from build123d import *

# Parameters (mm, degrees)
SKETCH2_W             = 39.3827
SKETCH2_H             = 7.62
BOSS_EXTRUDE2_DEPTH   = 4.445
BOSS_EXTRUDE2_2_DEPTH = 4.445
BOSS_EXTRUDE3_DEPTH   = 2.54
BOSS_EXTRUDE4_DEPTH   = 44.45
CUT_EXTRUDE3_REACH    = 78.845
SKETCH5_R             = 2.54
SKETCH5_R_2           = 1.0668
CUT_EXTRUDE5_DEPTH    = 41.91
CUT_EXTRUDE7_START    = 2.54
SKETCH7_W             = 22.974442495
SKETCH7_H             = 3.048
CUT_EXTRUDE7_DEPTH    = 16.51
CUT_EXTRUDE8_DEPTH    = 22.974442495


with BuildPart() as part:
    # Sketch2 → Boss-Extrude2 (new body)
    with BuildSketch(Plane(origin=(0, 0, 0), x_dir=(1, 0, 0), z_dir=(0, 1, 0))):
        with Locations((19.69135, 3.81)):
            Rectangle(SKETCH2_W, SKETCH2_H)
    extrude(amount=BOSS_EXTRUDE2_DEPTH)



with BuildPart() as body_2:
    # Sketch2 → Boss-Extrude2 2 (new body)
    with BuildSketch(Plane(origin=(0, 0, 0), x_dir=(1, 0, 0), z_dir=(0, 1, 0))):
        with Locations((19.69135, 72.39)):
            Rectangle(SKETCH2_W, SKETCH2_H)
    extrude(amount=BOSS_EXTRUDE2_2_DEPTH)


with BuildPart() as part_1:
    add(part.part)

    add(body_2.part)  # Boss-Extrude3 merges body 2
    # Sketch2<3> → Boss-Extrude3 (add)
    with BuildSketch(Plane(origin=(0, 0, 0), x_dir=(1, 0, 0), z_dir=(0, 1, 0))):
        with BuildLine():
            Line((0, 34.29), (0, 7.62))
            Line((0, 7.62), (39.3827, 7.62))
            Line((39.3827, 7.62), (39.3827, 68.58))
            Line((39.3827, 68.58), (0, 68.58))
            Line((0, 68.58), (0, 41.91))
            ThreePointArc((0, 41.91), (3.81, 38.1), (0, 34.29))
        make_face()
    extrude(amount=BOSS_EXTRUDE3_DEPTH)

    # Sketch2<8> → Boss-Extrude4 (add)
    with BuildSketch(Plane(origin=(0, 0, 0), x_dir=(1, 0, 0), z_dir=(0, 1, 0))):
        Polygon((8.533414456, 33.02), (8.533414456, 38.1), (8.533414456, 43.18), (16.153414456, 43.18), (31.507856951, 43.18), (31.507856951, 48.768), (6.107856951, 48.768), (6.107856951, 38.1), (6.107856951, 27.432), (31.507856951, 27.432), (31.507856951, 33.02), (16.153414456, 33.02), align=None)
    extrude(amount=BOSS_EXTRUDE4_DEPTH)

    # Cut-Extrude3: up to this face of the body (flat: up to its plane)
    cut_extrude3_end = Plane(part_1.part.faces().sort_by_distance((18.807856951, 23.495, -27.432))[0])
    # Sketch5 → Cut-Extrude3 (cut, up to the picked face)
    with BuildSketch(Plane(origin=(0, 0, -48.768), x_dir=(-1, 0, 0), z_dir=(0, 0, -1)), mode=Mode.PRIVATE) as cut_extrude3_sk1:
        with Locations((-13.727856951, 30.226)):
            Circle(SKETCH5_R)
    cut_extrude3_tool1 = split(extrude(cut_extrude3_sk1.sketch, amount=-CUT_EXTRUDE3_REACH, mode=Mode.PRIVATE), bisect_by=cut_extrude3_end, keep=Keep.BOTH, mode=Mode.PRIVATE)
    # Sketch5 → Cut-Extrude3 (cut, up to the picked face)
    with BuildSketch(Plane(origin=(0, 0, -48.768), x_dir=(-1, 0, 0), z_dir=(0, 0, -1)), mode=Mode.PRIVATE) as cut_extrude3_sk2:
        with Locations((-13.727856951, 24.6888)):
            Circle(SKETCH5_R_2)
    cut_extrude3_tool2 = split(extrude(cut_extrude3_sk2.sketch, amount=-CUT_EXTRUDE3_REACH, mode=Mode.PRIVATE), bisect_by=cut_extrude3_end, keep=Keep.BOTH, mode=Mode.PRIVATE)
    add(cut_extrude3_tool1.solids().sort_by(Axis((13.727857, 30.226, -48.768), (0, 0, 1)))[0], mode=Mode.SUBTRACT)
    add(cut_extrude3_tool2.solids().sort_by(Axis((13.727857, 24.6888, -48.768), (0, 0, 1)))[0], mode=Mode.SUBTRACT)

    # Sketch6 → Cut-Extrude5 (cut)
    with BuildSketch(Plane(origin=(0, 44.45, 0), x_dir=(1, 0, 0), z_dir=(0, 1, 0))):
        with BuildLine():
            Line((31.507856951, 29.125333333), (31.507856951, 27.432))
            Line((31.507856951, 27.432), (29.814523617, 27.432))
            ThreePointArc((29.814523617, 27.432), (31.0118911, 27.927965851), (31.507856951, 29.125333333))
        make_face()
        with BuildLine():
            Line((7.801190284, 48.768), (6.107856951, 48.768))
            Line((6.107856951, 48.768), (6.107856951, 47.074666667))
            ThreePointArc((6.107856951, 47.074666667), (6.603822801, 48.272034149), (7.801190284, 48.768))
        make_face()
        with BuildLine():
            Line((6.107856951, 29.125333333), (6.107856951, 27.432))
            Line((6.107856951, 27.432), (7.801190284, 27.432))
            ThreePointArc((7.801190284, 27.432), (6.603822801, 27.927965851), (6.107856951, 29.125333333))
        make_face()
        with BuildLine():
            Line((29.814523617, 48.768), (31.507856951, 48.768))
            Line((31.507856951, 48.768), (31.507856951, 47.074666667))
            ThreePointArc((31.507856951, 47.074666667), (31.0118911, 48.272034149), (29.814523617, 48.768))
        make_face()
    extrude(amount=-CUT_EXTRUDE5_DEPTH, mode=Mode.SUBTRACT)

    # Sketch7 → Cut-Extrude7 (cut)
    with BuildSketch(Plane(origin=(0, 2.54, 0), x_dir=(1, 0, 0), z_dir=(0, 1, 0)).offset(CUT_EXTRUDE7_START)):
        with Locations((20.020635704, 44.704)):
            Rectangle(SKETCH7_W, SKETCH7_H)
        with Locations((20.020635704, 31.496)):
            Rectangle(SKETCH7_W, SKETCH7_H)
    extrude(amount=CUT_EXTRUDE7_DEPTH, mode=Mode.SUBTRACT)

    # Sketch8 → Cut-Extrude8 (cut)
    with BuildSketch(Plane(origin=(31.507856951, 0, 0), x_dir=(0, 0, -1), z_dir=(1, 0, 0))):
        Polygon((33.02, 2.54), (29.972, 5.08), (33.02, 5.08), align=None)
        Polygon((43.18, 2.54), (46.228, 5.08), (43.18, 5.08), align=None)
    extrude(amount=-CUT_EXTRUDE8_DEPTH, mode=Mode.SUBTRACT)


solid = part_1.part
Geometry check sheet. Reference: the model listing, model coordinates, mm. A direction names the side the tool comes from. Give positions to 0.01 mm unless a question says otherwise; leave off trailing zeros. Order: outer loops, then holes, each group sorted by start corner. A loop starts at its lowest first (then second) coordinate and runs counter-clockwise, first axis right, second up. Notation, with made-up numbers: (47.5, 27) - (59.5, 27) arc R23 cw to (59.5, 43) - close; hole circle Ø2 at (-5.75, 61). An arc over 180 degrees is marked (long way). Use one line per item in the form item = value.
1) Sectioned sample at C-C (y = 15.5). Record the boundary of the cut face in (x, z), and give its area (3 significant figures).
Working result:
outline = (6.11, -47.07) arc R1.69 ccw to (7.8, -48.77) - (29.81, -48.77) arc R1.69 ccw to (31.51, -47.07) - (31.51, -46.23) - (8.53, -46.23) - (8.53, -29.97) - (31.51, -29.97) - (31.51, -29.13) arc R1.69 ccw to (29.81, -27.43) - (7.8, -27.43) arc R1.69 ccw to (6.11, -29.13) - close
area = 166 mm^2
2) Depth check by flat-ended pin: pin 1 Ø1.9 at (x, y) = (13.73, 24.69) entering from +Z; pin 2 Ø2.5 at (x, z) = (22.5, -5) entering from +Y (3 decimals); pin 3 Ø6 at (x, y) = (13.73, 30.23) entering from +Z; pin 4 Ø4.5 at (y, z) = (13, -31.5) entering from +X. Enter the tip coordinate at first touch or a pass-through.
Working result:
pin_1 = through
pin_2 = 4.445
pin_3 = -27.43
pin_4 = 31.51
3) Sectioned sample at B-B (z = -31). Record the boundary of the cut face in (x, y), and give its area (3 significant figures).
Working result:
outline = (0, 0) - (39.38, 0) - (39.38, 2.54) - (31.51, 2.54) - (31.51, 4.22) - (8.53, 4.22) - (8.53, 21.59) - (31.51, 21.59) - (31.51, 44.45) - (6.11, 44.45) - (6.11, 2.54) - (0, 2.54) - close; hole circle Ø5.08 at (13.73, 30.23); hole circle Ø2.13 at (13.73, 24.69)
area = 742 mm^2
4) Sectioned sample at A-A (x = 33). Record the boundary of the cut face in (y, z) (3 decimals), and give its area (3 significant figures).
Working result:
outline = (0, -76.2) - (4.445, -76.2) - (4.445, -68.58) - (2.54, -68.58) - (2.54, -7.62) - (4.445, -7.62) - (4.445, 0) - (0, 0) - close
area = 223 mm^2
5) Material ranges on probe 1 along Z at (x, y) = (20, 35.5); probe 2 along Z at (x, y) = (18, 20); probe 3 along Y at (x, z) = (8, -17.5), recorded low to high. Write a range as from..to.
Working result:
probe_1 = -48.77..-43.18, -33.02..-27.43
probe_2 = -48.77..-46.23, -29.97..-27.43
probe_3 = 0..2.54
6) Draft check along Z on faces 5 (the face through (19, 4.445, -72)), 6 (the face through (20.18, 3.79, -31.52)), 7 (the face through (20, 33, -43.18)), 8 (the face through (19, 2, 0)). Enter one of: released by +Z, released by -Z, zero draft, split by the parting line, or undercut.
Working result:
face_5 = zero draft
face_6 = undercut
face_7 = undercut
face_8 = released by +Z
7) Access from +Z, -Z, +X, -X, +Y, -Y to the whole of each face (thin tool, end or side, straight path). Record for faces 1 (the face through (19, 4.445, -4)), 2 (the face through (19, 3, -7.62)), 3 (the face through (14.278, 27.746, -30.265)), 4 (the face through (20, 21.59, -45)).
Working result:
face_1 = +Z, +X, -X, +Y
face_2 = +X, -X, +Y
face_3 = +Z, -Z
face_4 = +X
